from build123d import *

# Parameters (mm, degrees)
F1_DEPTH = 6
F0_W     = 27
F0_H     = 47
F0_R     = 9.5
F2_DEPTH = 22
F3_DEPTH = 22


with BuildPart() as f1:
    # F0 (on Top) → F1 (new body)
    with BuildSketch(Plane.XY):
        with BuildLine():
            Line((2, 9.6277186767), (2, 15.3722813233))
            ThreePointArc((2, 15.3722813233), (0, 16), (-2, 15.3722813233))
            Line((-2, 15.3722813233), (-2, 9.6277186767))
            ThreePointArc((-2, 9.6277186767), (0, 9), (2, 9.6277186767))
        make_face()
    extrude(amount=F1_DEPTH)

    # F0 (on Top) → F2 (join)
    with BuildSketch(Plane.XY):
        Rectangle(F0_W, F0_H)
        with Locations((0, 12.5)):
            Circle(F0_R, mode=Mode.SUBTRACT)
        with Locations((0, 12.5)):
            Circle(F0_R)
        with BuildLine():
            ThreePointArc((2, 15.3722813233), (3.1024184115, 14.1201851746), (3.5, 12.5))
            ThreePointArc((3.5, 12.5), (3.1024184115, 10.8798148254), (2, 9.6277186767))
            ThreePointArc((2, 9.6277186767), (0, 9), (-2, 9.6277186767))
            ThreePointArc((-2, 9.6277186767), (-3.5, 12.5), (-2, 15.3722813233))
            ThreePointArc((-2, 15.3722813233), (0, 16), (2, 15.3722813233))
        make_face(mode=Mode.SUBTRACT)
        with BuildLine():
            Line((-2, 9.6277186767), (-2, 15.3722813233))
            ThreePointArc((-2, 15.3722813233), (-3.5, 12.5), (-2, 9.6277186767))
        make_face()
        with BuildLine():
            ThreePointArc((2, 9.6277186767), (3.1024184115, 10.8798148254), (3.5, 12.5))
            ThreePointArc((3.5, 12.5), (3.1024184115, 14.1201851746), (2, 15.3722813233))
            Line((2, 15.3722813233), (2, 9.6277186767))
        make_face()
    extrude(amount=-F2_DEPTH)

    # F0 (on Top) → F3 (join)
    with BuildSketch(Plane.XY):
        with BuildLine():
            Line((2, 9.6277186767), (2, 15.3722813233))
            ThreePointArc((2, 15.3722813233), (0, 16), (-2, 15.3722813233))
            Line((-2, 15.3722813233), (-2, 9.6277186767))
            ThreePointArc((-2, 9.6277186767), (0, 9), (2, 9.6277186767))
        make_face()
    extrude(amount=-F3_DEPTH)


solid = f1.part
Part model, mm, in its own coordinate system. A direction names the side the tool comes from. Coordinates: 2 decimals unless noted, no trailing zeros. Write each loop counter-clockwise with the first axis right and the second up, starting at its lowest first coordinate (ties: lowest second). Pieces come first, ordered by that corner, then holes. Notation, with made-up numbers: (29, 25) - (45, 25) arc R8 ccw to (45, 39) - close; hole circle Ø3 at (-38.5, -6.5). An arc over 180 degrees is marked (long way). Put each result on its own line as item: value.
1. Band-saw the part on A-A (z = 0.5). Write the cut outline in (x, y), then the cut area to 3 significant figures.
Final values:
outline: (-2, 9.63) arc R3.5 ccw to (2, 9.63) - (2, 15.37) arc R3.5 ccw to (-2, 15.37) - close
area: 26.4 mm²
2. Band-saw the part on B-B (x = 9.75). Write the cut outline in (y, z).
Final values:
outline: (-23.5, -22) - (23.5, -22) - (23.5, 0) - (-23.5, 0) - close
3. Probe line 1 along Z through (x, y) = (-1.5, -10); line 2 along X through (y, z) = (10, 2.5); line 3 along Y through (x, z) = (1, 3.75). List the from-to ranges inside material, lowest first. Write a range as [from, to].
Final values:
line 1: z = [-22, 0]
line 2: x = [-2, 2]
line 3: y = [9.15, 15.85]
4. 3-axis set-ups, long thin cutter, end or side, ignore diameter. For faces 1 (the cylindrical face through (0, 9, 3)), 2 (the cylindrical face through (0, 16, 3)), 3 (the flat face through (2, 12, 3)), 4 (the flat face through (-2, 13, 3)): which of +Z, -Z, +X, -X, +Y, -Y reach the whole face in a straight line?
Final values:
face 1: +Z, -Y
face 2: +Z, +Y
face 3: +Z, +X, +Y, -Y
face 4: +Z, -X, +Y, -Y
5. Flat gauge pin, fed straight in: pin 1 Ø4.5 at (y, z) = (13.5, 2.5) entering from +X. Where does the tip first touch, or does it go through?
Final values:
pin 1: stops at x = 2
